```python
from build123d import *

# Parameters (mm, degrees)
SKETCH1_R           = 8
BOSS_EXTRUDE1_DEPTH = 30
SKETCH2_R           = 20
BOSS_EXTRUDE2_DEPTH = 5
CHAMFER1_SIZE       = 2
SKETCH3_R           = 2.5
CUT_EXTRUDE1_DEPTH  = 71.887234394
CIRPATTERN1_COUNT   = 4


with BuildPart() as part:
    # Sketch1 → Boss-Extrude1 (new, symmetric)
    with BuildSketch(Plane(origin=(0, 0, 0), x_dir=(1, 0, 0), z_dir=(0, 1, 0))):
        with Locations(Location((0, 0, 0), (0, 0, 270))):
            Circle(SKETCH1_R)
    extrude(amount=BOSS_EXTRUDE1_DEPTH, both=True)

    # Sketch2 → Boss-Extrude2 (add)
    with BuildSketch(Plane(origin=(0, 30, 0), x_dir=(1, 0, 0), z_dir=(0, 1, 0))):
        with Locations(Location((0, 0, 0), (0, 0, 270))):
            Circle(SKETCH2_R)
    extrude(amount=BOSS_EXTRUDE2_DEPTH)

    # Chamfer1
    chamfer1_edges = [part.edges().sort_by_distance(p)[0] for p in [
        (0, 35, -20),
    ]]
    chamfer(chamfer1_edges, length=CHAMFER1_SIZE)

    # Sketch3 → Cut-Extrude1 (cut, through all)
    with BuildSketch(Plane(origin=(0, 35, 0), x_dir=(1, 0, 0), z_dir=(0, 1, 0))):
        with Locations(Location((0, 13, 0), (0, 0, 270))):
            Circle(SKETCH3_R)
    cut_extrude1 = extrude(amount=-CUT_EXTRUDE1_DEPTH, mode=Mode.SUBTRACT)

    # CirPattern1: Cut-Extrude1 ×4 about axis
    cirpattern1_axis = Axis((0, 0, 0.25570417), (0, 1, 0))
    for i in range(1, CIRPATTERN1_COUNT):
        add(cut_extrude1.rotate(cirpattern1_axis, i * 360 / CIRPATTERN1_COUNT), mode=Mode.SUBTRACT)

    # Mirror1: part across plane


with BuildPart() as part_1:
    add(part.part)
    add(part.part.mirror(Plane.ZX))


solid = part_1.part
```
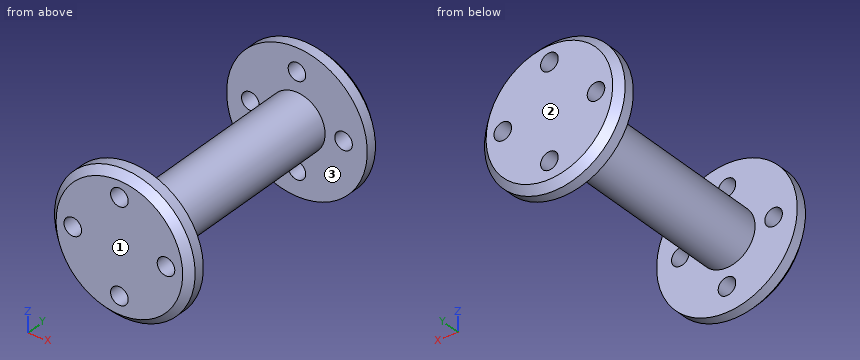
Part model, mm, in its own coordinate system. Face numbers are marked on the shaded views. Coordinates: 2 decimals unless noted, no trailing zeros. Loops run counter-clockwise (first coordinate to the right, second up) from the corner with the lowest first, then second, coordinate; pieces in that order, holes last. Notation, with made-up numbers: (72, 24.5) - (127, 24.5) arc R28 ccw to (127, 43.5) - close; hole circle Ø6 at (7, 72.5). An arc over 180 degrees is marked (long way). Write item = value, one per line. Start each with the question number.
Item 1: Cut at A-A, the plane x = 0. State how many separate pieces and enclosed holes the cut face has, and give its area (3 significant figures).
Item 2: Flat gauge pins, fed straight in: pin 1 Ø2 at (x, y) = (4, 3.5) entering from -Z; pin 2 Ø1.5 at (x, y) = (4.5, -17.5) entering from -Z; pin 3 Ø5 at (y, z) = (16.5, -9.5) entering from -X; pin 4 Ø3 at (x, z) = (0, 13.51) entering from -Y. Where does each tip first touch, or does it go through?
Item 3: Mould opens along Y. For the marked faces 1, 2 and 3 say: released by +Y, released by -Y, zero draft, split by the parting line, or undercut.
Item 4: Wall check: L1, parallel to Y at x = -10.5, z = 4; L2, parallel to X at y = -33.25, z = -13; L3, parallel to X at y = -29.5, z = -1. Give the ranges that are in metal, low to high. Write a range as from..to.
Item 5: Cut at C-C, the plane y = 15. Give the cut face in (x, z).
The answers:
q1.separate_pieces = 5
q1.enclosed_holes = 0
q1.area = 1,250 mm2
q2.pin_1 = -7.42
q2.pin_2 = -7.07
q2.pin_3 = -3.87
q2.pin_4 = through
q3.face_1 = released by -Y
q3.face_2 = released by +Y
q3.face_3 = undercut
q4.L1 = -35..-30, 30..35
q4.L2 = -14.87..-2.5, 2.5..14.87
q4.L3 = -7.94..7.94
q5.outline = circle Ø16 at (0, 0)
